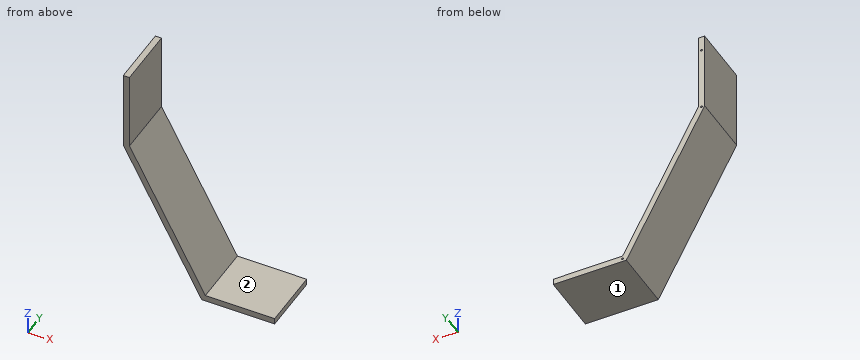
Autodesk Inventor part; units mm, degrees
ref_plane "YZ Plane" through (0, 0, 0) normal (1, 0, 0) x (0, 1, 0)
ref_plane "XZ Plane" through (0, 0, 0) normal (0, 1, 0) x (-1, 0, 0)
ref_plane "XY Plane" through (0, 0, 0) normal (0, 0, 1) x (1, 0, 0)
sketch "スケッチ1" plane through (0, 0, 0) normal (0, 1, 0) x (-1, 0, 0)
  line L0 (0, 0) -> (8, 0)
  line L1 (8, 0) -> (8, -90)
  line L2 (8, -90) -> (0, -90)
  line L3 (0, -90) -> (0, 0)
  line L4 (-94, -275) -> (-189, -275)
  line L5 (-189, -275) -> (-189, -283)
  line L6 (-189, -283) -> (-94, -283)
  line L7 (-94, -283) -> (-94, -275)
  line L8 (8, -90) -> (-94, -283)
  line L9 (0, -88.016) -> (-98.8205, -275)
  line L10 (8, 0) -> (0, 0)
  line L11 (0, 0) -> (0, 15)
  line L12 (0, 15) -> (8, 15)
  line L13 (8, 15) -> (8, 0)
  dimension "d0" = 8
  dimension "d1" = 90
  dimension "d4" = 8
  dimension "d5" = 185
  dimension "d6" = 94
  dimension "d7" = 8
  dimension "d20" = 95
  dimension "d21" = 15
extrude "押し出し1" add sketch "スケッチ1" along normal blind 80
sketch "スケッチ2" plane through (0, 80, 0) normal (0, 1, 0) x (1, 0, 0)
  line L0 (0, -15) -> (0, 88.016)
  point P0 (-4, 5)
  point P1 (-4, 90)
  point P2 (99, 279)
  point P3 (-4, 0)
  dimension "d8" = 5
  dimension "d9" = 85
  dimension "d11" = 189
  dimension "d12" = 103
  dimension "d22" = 4
hole "穴1" at (-4, 80, -5) at (-4, 80, -90) at (99, 80, -279) direction (0, -1, 0) diameter 2.459 depth 8.8 tip angle 118
properties part number "右仕切り"
Geometry check sheet. Reference: the model listing, model coordinates, mm. Face numbers are marked on the shaded views. A direction names the side the tool comes from. Round coordinates to 2 decimals unless told otherwise and drop trailing zeros. Order: outer loops, then holes, each group sorted by start corner. A loop starts at its lowest first (then second) coordinate and runs counter-clockwise, first axis right, second up. Notation, with made-up numbers: (11, 3.5) - (66, 3.5) arc R9 cw to (66, 11.5) - close; hole circle Ø9 at (61.5, 64). An arc over 180 degrees is marked (long way). Use a Markdown table: item, result. Add a question column.
(1) Depth check by flat-ended pin: pin 1 (1.5 mm diameter, centred on y = 69.5, z = -56, fed in from +X); pin 2 (4 mm diameter, centred on y = 59, z = -177, fed in from +X); pin 3 (12 mm diameter, centred on x = 156, y = 21.5, fed in from +Z). Enter the tip coordinate at first touch or a pass-through.
(2) Sectioned sample at A-A, the plane y = 7. Enter the section's corners in (x, z).
(3) Sectioned sample at C-C, the plane x = 137.5. Enter the section's corners in (y, z), and give its area (3 significant figures).
(4) Material ranges on line 1 along Z through (x, y) = (-4, 76.5); line 2 along X through (y, z) = (75, -5); line 3 along Z through (x, y) = (99, 76), recorded low to high. Write a range as [from, to].
(5) Tool access check on the marked faces 1 and 2. Record the directions out of +Z, -Z, +X, -X, +Y, -Y that give a thin tool (end or side, any length) a straight path to the whole face; none if there is none.
(6) Sectioned sample at B-B, the plane z = -20. Enter the section's corners in (x, y).
Answers below:
| question | item | result |
|---|---|---|
| 1 | pin 1 | x = 0 |
| 1 | pin 2 | x = 48.08 |
| 1 | pin 3 | z = -275 |
| 2 | outline | (-8, -90) - (94, -283) - (189, -283) - (189, -275) - (98.82, -275) - (0, -88.02) - (0, 15) - (-8, 15) - close |
| 3 | outline | (0, -283) - (80, -283) - (80, -275) - (0, -275) - close |
| 3 | area | 640 mm² |
| 4 | line 1 | [-97.57, -91.23], [-88.77, -6.23], [-3.77, 15] |
| 4 | line 2 | [-8, -5.23], [-2.77, 0] |
| 4 | line 3 | [-283, -280.23], [-277.77, -275] |
| 5 | face 1 | -Z, +X, -X, +Y, -Y |
| 5 | face 2 | +Z, +X, +Y, -Y |
| 6 | outline | (-8, 0) - (0, 0) - (0, 80) - (-8, 80) - close |
